Source: CAD feature listing. Evaluate the final solid. Frame: model axes, mm. A direction names the side the tool comes from. Give positions to 0.01 mm unless a question says otherwise; leave off trailing zeros. Order: outer loops, then holes, each group sorted by start corner. A loop starts at its lowest first (then second) coordinate and runs counter-clockwise, first axis right, second up. Notation, with made-up numbers: (82, 44) - (118, 44) arc R13 cw to (118, 53) - close; hole circle Ø3 at (85.5, 38.25). An arc over 180 degrees is marked (long way). Write each question's results on one line, items separated by ' | '. Start each with the question number.
Item 1: Set-up query: faces 4 (the flat face through (0, -47, -4.5)), 5 (the cylindrical face through (-0.651, -32.43, -11.957)), 6 (the cylindrical face through (0, 55, -1)). Return all of +Z, -Z, +X, -X, +Y, -Y with unobstructed straight access to the full face (end or side cutting, diameter ignored); none if empty.
Item 2: Section D-D on z = -8.5. Output: boundary loops of the cut face in (x, y), and give its area (3 significant figures).
Item 3: Contact query for flat-ended pins moving along their axis: pin 1 Ø12 at (x, y) = (-9.5, 20) entering from +Z; pin 2 Ø3 at (y, z) = (-9, -8) entering from -X; pin 3 Ø1 at (x, y) = (2, 42) entering from +Z. Output: stop coordinate, or through.
Item 4: Section A-A on y = 4.5. Output: boundary loops of the cut face in (x, z), and give its area (3 significant figures).
Item 5: Section B-B on x = 19.5. Output: boundary loops of the cut face in (y, z).
Item 6: Mould query, pull axis X, two halves, no side actions, for faces 1 (the flat face through (3.3, -37.5, -6.9)), 2 (the cylindrical face through (17.517, 4.24, -20.543)), 3 (the cylindrical face through (-13.887, 25.65, -10.648)). Classes: released by +X, released by -X, zero draft, split by the parting line, or undercut.
Item 7: Line query: line 1 along X through (y, z) = (44.5, -20.3); line 2 along Y through (x, z) = (19.5, -20.5); line 3 along Y through (x, z) = (5, 6). Output: solid intervals per line, ascending.
Item 8: Section C-C on y = 28. Output: boundary loops of the cut face in (x, z), and give its area (3 significant figures).
Autodesk Inventor part; units mm, degrees
ref_plane "YZ Plane" through (0, 0, 0) normal (1, 0, 0) x (0, 1, 0)
ref_plane "XZ Plane" through (0, 0, 0) normal (0, 1, 0) x (-1, 0, 0)
ref_plane "XY Plane" through (0, 0, 0) normal (0, 0, 1) x (1, 0, 0)
sketch "Esquisse1" plane through (0, 0, 0) normal (0, 1, 0) x (-1, 0, 0)
  circle A0 centre (0, 0) radius 18.25
  line L0 (-15, 0) -> (15, 0)
  line L1 (15, 0) -> (15, -20.05)
  line L2 (15, -20.05) -> (-15, -20.05)
  line L3 (-15, -20.05) -> (-15, 0)
  line L4 (-23.5, -21.05) -> (23.5, -21.05)
  line L5 (23.5, -21.05) -> (23.5, -20.05)
  line L6 (23.5, -20.05) -> (-23.5, -20.05)
  line L7 (-23.5, -20.05) -> (-23.5, -21.05)
  dimension "d0" = 36.5
  dimension "d1" = 30
  dimension "d2" = 15
  dimension "d3" = 1
  dimension "d4" = 47
  dimension "d5" = 23.5
  dimension "d6" = 39.3
extrude "Extrusion1" add sketch "Esquisse1" along normal blind 1
sketch "Esquisse2" plane through (0, 1, 0) normal (0, 1, 0) x (1, 0, 0)
  arc A0 (-15, 10.3953) -> (15, 10.3953) centre (0, 0) ccw
  circle A1 centre (0, 0) radius 17.5
  dimension "d9" = 35
extrude "Extrusion2" add sketch "Esquisse2" along normal blind 50
sketch "Esquisse3" plane through (0, 0, 0) normal (0, -1, 0) x (1, 0, 0)
  arc A0 (15, -10.3953) -> (-15, -10.3953) centre (0, 0) ccw
  circle A1 centre (0, 0) radius 17.5
  dimension "d12" = 35
extrude "Extrusion3" add sketch "Esquisse3" along normal blind 27.5
sketch "Esquisse4" plane through (0, 1, 0) normal (0, 1, 0) x (1, 0, 0)
  line L0 (-23.5, 21.05) -> (23.5, 21.05)
  line L1 (23.5, 21.05) -> (23.5, 20.05)
  line L2 (23.5, 20.05) -> (-23.5, 20.05)
  line L3 (-23.5, 20.05) -> (-23.5, 21.05)
extrude "Extrusion4" add sketch "Esquisse4" along normal blind 48
sketch "Esquisse5" plane through (0, -27.5, 0) normal (0, -1, 0) x (1, 0, 0)
  circle A0 centre (0, 0) radius 17.5
  line L0 (0, 0) -> (0, -17.5)
  circle A1 centre (0, -7) radius 5
  dimension "d17" = 7
  dimension "d18" = 10
extrude "Extrusion5" add sketch "Esquisse5" along normal blind 10 contours A1 L0 | L0 A1
sketch "Esquisse6" plane through (0, -37.5, -7) normal (0, -1, 0) x (1, 0, 0)
  circle A0 centre (0, 0) radius 5
  circle A1 centre (0, 0) radius 3
  point P0 (0, 7)
  dimension "d21" = 6
extrude "Extrusion6" add sketch "Esquisse6" along normal blind 15 contours A1
sketch "Esquisse7" plane through (0, -52.5, -7) normal (0, -1, 0) x (1, 0, 0)
  circle A0 centre (0, 0) radius 3
  line L0 (-1.6583, 2.5) -> (1.6583, 2.5)
  line L1 (1.6583, 2.5) -> (1.6583, 0)
  line L2 (1.6583, 0) -> (-1.6583, 0)
  line L3 (-1.6583, 0) -> (-1.6583, 2.5)
  arc A1 (1.6583, 2.5) -> (-1.6583, 2.5) centre (0, 0) ccw
  arc A2 (-1.6583, 2.5) -> (1.6583, 2.5) centre (0, 0) ccw
  point P0 (0, 7)
  dimension "d27" = 5.5
extrude "Extrusion7" cut sketch "Esquisse7" against normal blind 12 contours L0 A0
sketch "Esquisse8" plane through (0, 51, 0) normal (0, 1, 0) x (1, 0, 0)
  circle A0 centre (0, 0) radius 17.5
  circle A1 centre (0, 0) radius 5
  dimension "d28" = 10
extrude "Extrusion8" add sketch "Esquisse8" along normal blind 3 contours A1
sketch "Esquisse9" plane through (0, 54, 0) normal (0, 1, 0) x (1, 0, 0)
  circle A0 centre (0, 0) radius 5
  circle A1 centre (0, 0) radius 1
  dimension "d31" = 2
extrude "Extrusion9" add sketch "Esquisse9" along normal blind 3 contours A1
sketch "Esquisse10" plane through (23.5, 0, -21.05) normal (0, 0, -1) x (-1, 0, 0)
  line L0 (0, 0) -> (47, 0)
  line L1 (47, 0) -> (47, 49)
  line L2 (0, 49) -> (47, 49)
  line L3 (0, 0) -> (0, 49)
  line L4 (4, 44.5) -> (43, 44.5)
  line L5 (43, 44.5) -> (43, 4.5)
  line L6 (43, 4.5) -> (4, 4.5)
  line L7 (4, 4.5) -> (4, 44.5)
  point P0 (23.5, 0)
  dimension "d34" = 39
  dimension "d35" = 47
  dimension "d36" = 4
  dimension "d37" = 40
  dimension "d38" = 49
  dimension "d39" = 4.5
hole "Perçage1" at (19.5, 44.5, -21.05) at (-19.5, 44.5, -21.05) at (-19.5, 4.5, -21.05) at (19.5, 4.5, -21.05) direction (0, 0, 1) diameter 4 end through all
equation "\"d36\" = -0.5 * d34 + 0.5 * d35"
equation "\"d39\" = -0.5 * d37 + 0.5 * d38"
properties part number "mfa_970d471"
Evaluation:
1) face 4: +Z, +X, -X, -Y | face 5: -Y | face 6: +Y
2) outline: (-16.15, 0) - (-15.3, 0) - (-15.3, -27.5) - (-4.77, -27.5) - (-4.77, -37.5) - (-2.6, -37.5) - (-2.6, -52.5) - (2.6, -52.5) - (2.6, -37.5) - (4.77, -37.5) - (4.77, -27.5) - (15.3, -27.5) - (15.3, 0) - (16.15, 0) - (16.15, 1) - (15.3, 1) - (15.3, 51) - (-15.3, 51) - (-15.3, 1) - (-16.15, 1) - close | area: 2,580 mm^2
3) pin 1: stops at z = 17.15 | pin 2: stops at x = -16.25 | pin 3: stops at z = 17.44
4) outline: (-23.5, -21.05) - (-21.5, -21.05) - (-21.5, -20.05) - (-23.5, -20.05) - close; (-17.5, -21.05) - (17.5, -21.05) - (17.5, -20.05) - (-17.5, -20.05) - close; circle Ø35 at (0, 0); (21.5, -21.05) - (23.5, -21.05) - (23.5, -20.05) - (21.5, -20.05) - close | area: 1,000 mm^2
5) outline: (0, -21.05) - (2.5, -21.05) - (2.5, -20.05) - (0, -20.05) - close; (6.5, -21.05) - (42.5, -21.05) - (42.5, -20.05) - (6.5, -20.05) - close; (46.5, -21.05) - (49, -21.05) - (49, -20.05) - (46.5, -20.05) - close
6) face 1: zero draft | face 2: undercut | face 3: split by the parting line
7) line 1: x = -23.5 to -21.5, -17.5 to 17.5, 21.5 to 23.5 | line 2: y = 0 to 2.5, 6.5 to 42.5, 46.5 to 49 | line 3: y = -27.5 to 51
8) outline: (-23.5, -21.05) - (23.5, -21.05) - (23.5, -20.05) - (-23.5, -20.05) - close; circle Ø35 at (0, 0) | area: 1,010 mm^2
